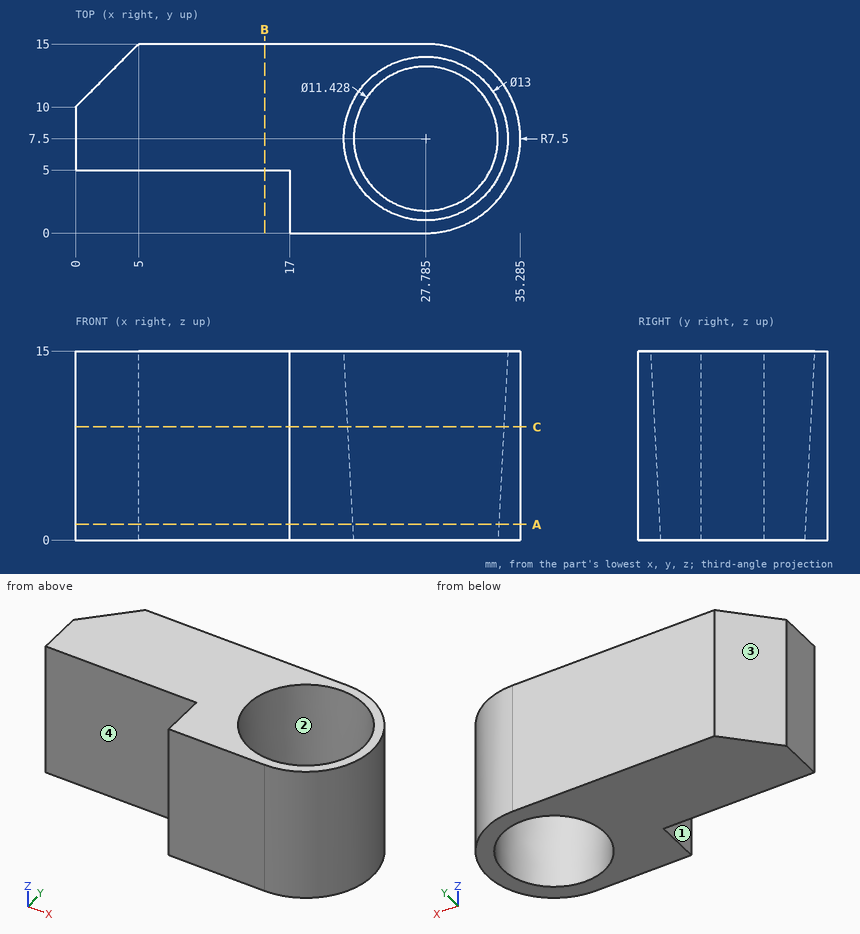
Job drawing, mm, ordinate dimensions from the low corner. One solid piece. Give positions to 0.01 mm unless a question says otherwise; leave off trailing zeros. Loops run counter-clockwise (first coordinate to the right, second up) from the corner with the lowest first, then second, coordinate; pieces in that order, holes last. Notation, with made-up numbers: (-4.5, 26.25) -> (27.5, 26.25) arc R21 cw to (27.5, 33.25) -> close; hole circle Ø10 at (20.5, 75). An arc over 180 degrees is marked (long way). Use a Markdown table: item, result. Add a question column.
(1) Slice it at B-B on x = 15. List the corners of the cut face in (y, z), and give its area (3 significant figures).
(2) Wall check: line 1 along Y through (x, z) = (9.5, 3.25); line 2 along X through (y, z) = (8, 7.5); line 3 along X through (y, z) = (7.5, 6) (1 decimal). Give the ranges that are in metal, low to high.
(3) Drop flat-ended pins along their axis: pin 1 Ø1 at (x, z) = (30.5, 10) entering from -Y (1 decimal); pin 2 Ø7.5 at (x, z) = (7.5, 4) entering from -Y; pin 3 Ø8 at (x, z) = (29, 9.5) entering from +Y; pin 4 Ø3 at (y, z) = (1.5, 7.5) entering from +X (1 decimal). Give the stop position or say it passes through.
(4) Slice it at A-A on z = 1.25. List the corners of the cut face in (x, y) (1 decimal), and give its area (3 significant figures).
(5) Slice it at C-C on z = 9. List the corners of the cut face in (x, y) (1 decimal).
(6) Mould opens along Y. For the marked faces 1, 2, 3 and 4 say: +Y half, -Y half, draft (parallel to the pull), parting line (faces both ways), or undercut.
Filled sheet:
| question | item | result |
|---|---|---|
| 1 | outline | (5, 0) -> (15, 0) -> (15, 15) -> (5, 15) -> close |
| 1 | area | 150 mm2 |
| 2 | line 1 | 5 to 15 |
| 2 | line 2 | 0 to 21.7, 33.87 to 35.27 |
| 2 | line 3 | 0 to 21.8, 33.8 to 35.3 |
| 3 | pin 1 | y = 0.3 |
| 3 | pin 2 | y = 5 |
| 3 | pin 3 | y = 15 |
| 3 | pin 4 | x = 33.8 |
| 4 | outline | (0, 5) -> (17, 5) -> (17, 0) -> (27.8, 0) arc R7.5 ccw to (27.8, 15) -> (5, 15) -> (0, 10) -> close; hole circle Ø11.6 at (27.8, 7.5) |
| 4 | area | 303 mm2 |
| 5 | outline | (0, 5) -> (17, 5) -> (17, 0) -> (27.8, 0) arc R7.5 ccw to (27.8, 15) -> (5, 15) -> (0, 10) -> close; hole circle Ø12.4 at (27.8, 7.5) |
| 6 | face 1 | draft |
| 6 | face 2 | undercut |
| 6 | face 3 | +Y half |
| 6 | face 4 | -Y half |
